```python
from build123d import *

# Parameters (mm, degrees)
SKETCH_R  = 1
PAD_DEPTH = 6


with BuildPart() as part:
    # Sketch → Pad (new body)
    with BuildSketch(Plane.XZ):
        Polygon((0, 13), (0, 3), (1, 3), (1, 0), (2, 0), (2, 3), (9, 3), (9, 0), (10, 0), (10, 3), (18, 3), (18, 0), (19, 0), (19, 3), (20, 3), (20, 13), (17.5, 13), (3, 18), (0, 18), (0, 17.5), (3, 17.5), (16.05, 13), align=None)
        with Locations((5.5, 5.5)):
            Circle(SKETCH_R, mode=Mode.SUBTRACT)
        with Locations((14.5, 5.5)):
            Circle(SKETCH_R, mode=Mode.SUBTRACT)
    extrude(amount=PAD_DEPTH)


solid = part.part
```
Work out the finished part from the listing and answer in its coordinate system (mm). A direction names the side the tool comes from. Give positions to 0.01 mm unless a question says otherwise; leave off trailing zeros. Order: outer loops, then holes, each group sorted by start corner. A loop starts at its lowest first (then second) coordinate and runs counter-clockwise, first axis right, second up. Notation, with made-up numbers: M 47,34 L 95,34 A18 cw 95,54 Z; hole C -17,41 d5. An arc over 180 degrees is marked long. Return JSON: item names as keys, results as strings.
1) A tool of negligible diameter and unlimited length cuts with its end or side. For faces 1 (the flat face through (19.5, -3, 3)), 2 (the flat face through (19, -3, 13)), 3 (the flat face through (9, -3, 2)), from which of +Z, -Z, +X, -X, +Y, -Y can it reach the whole face along a straight path? Write none if from no direction.
Resolved:
{"face 1": "-Z, +X, +Y, -Y", "face 2": "+Z, +X, +Y, -Y", "face 3": "-Z, +Y, -Y"}
2) Straight lines are drawn through the part: line 1 along X through (y, z) = (-2.05, 2); line 2 along X through (y, z) = (-4.4, 6); line 3 along Z through (x, y) = (1.5, -5.25). For each, find the intervals that lie inside material, in ascending order. Write a range as [from, to].
Resolved:
{"line 1": "[1, 2], [9, 10], [18, 19]", "line 2": "[0, 4.63], [6.37, 13.63], [15.37, 20]", "line 3": "[0, 13], [17.5, 18]"}
3) Section A-A, the plane y = -4.9 is taken. Write down the section's boundary in (x, z).
Resolved:
{"outline": "M 0,3 L 1,3 L 1,0 L 2,0 L 2,3 L 9,3 L 9,0 L 10,0 L 10,3 L 18,3 L 18,0 L 19,0 L 19,3 L 20,3 L 20,13 L 17.5,13 L 3,18 L 0,18 L 0,17.5 L 3,17.5 L 16.05,13 L 0,13 Z; hole C 5.5,5.5 d2; hole C 14.5,5.5 d2"}
4) For a pull along X with two mould halves and no side action, classify faces 4 (the flat face through (1.5, -3, 0)), 5 (the flat face through (5, -3, 3)), 6 (the flat face through (14, -3, 3)), 7 (the flat face through (1, -3, 2)) as +X half, -X half, draft (parallel to the pull), parting line (faces both ways), or undercut.
Resolved:
{"face 4": "draft", "face 5": "undercut", "face 6": "undercut", "face 7": "-X half"}
5) Section C-C, the plane x = 14.5 is taken. Write down the section's boundary in (y, z).
Resolved:
{"outline": "M -6,3 L 0,3 L 0,4.5 L -6,4.5 Z; M -6,6.5 L 0,6.5 L 0,13 L -6,13 Z; M -6,13.53 L 0,13.53 L 0,14.03 L -6,14.03 Z"}
6) Section D-D, the plane x = 18.5 is taken. Write down the section's boundary in (y, z).
Resolved:
{"outline": "M -6,0 L 0,0 L 0,13 L -6,13 Z"}
7) Section B-B, the plane z = 1.5 is taken. Write down the section's boundary in (x, y).
Resolved:
{"outline": "M 1,-6 L 2,-6 L 2,0 L 1,0 Z; M 9,-6 L 10,-6 L 10,0 L 9,0 Z; M 18,-6 L 19,-6 L 19,0 L 18,0 Z"}
8) Each of these flat-tipped pins is pushed along its axis until it touches: pin 1 (0.9 mm diameter, centred on y = -3.5, z = 1.5, fed in from +X); pin 2 (0.9 mm diameter, centred on y = -2.5, z = 2, fed in from -X). Where does it stop, or does it pass through?
Resolved:
{"pin 1": "x = 19", "pin 2": "x = 1"}
